Work out the finished part from the listing and answer in its coordinate system (mm). Give positions to 0.01 mm unless a question says otherwise; leave off trailing zeros. Write each loop counter-clockwise with the first axis right and the second up, starting at its lowest first coordinate (ties: lowest second). Pieces come first, ordered by that corner, then holes.
1) Given pin 1 Ø1.5 at (x, z) = (13, -56.5) entering from +Y; pin 2 Ø2 at (x, y) = (12, -6) entering from +Z; pin 3 Ø5 at (x, y) = (2, -7) entering from -Z, each flat-ended and moving along its own axis, determine where each tip first touches the part or whether it passes through.
2) Straight lines are drawn through the part: probe 1 along X at (y, z) = (-20.5, -8); probe 2 along Y at (x, z) = (5, -39.5); probe 3 along X at (y, z) = (-23, -27.5). For each, find the intervals that lie inside material, in ascending order.
3) Find section B-B (y = -9.25). Determine the outline of the cut face in (x, z), plus the area to 3 significant figures.
4) Find section A-A (z = -16). Determine the outline of the cut face in (x, y).
```python
from build123d import *

# Parameters (mm, degrees)
F0_W         = 14.6878659725
F0_H         = 93.4034362435
F1_DEPTH     = 25.4
F2_R         = 5.08
F3_R         = 5.08
F4_T1_DEPTH  = 4.5278659725
F4_T3_DEPTH  = 15.24
F4_S7_W      = 5.08
F4_S7_H      = 5.08
F4_T8_DEPTH  = 5.08
F4_S13_W     = 5.08
F4_S13_H     = 5.08
F4_T14_DEPTH = 5.08
F4_S19_W     = 5.08
F4_S19_H     = 5.08
F4_T20_DEPTH = 5.08
F4_S25_W     = 5.08
F4_S25_H     = 5.08
F4_T26_DEPTH = 5.08
F4_T30_ANGLE = 90
F4_T32_ANGLE = 90
F4_T34_ANGLE = 90
F4_T36_ANGLE = 90


# Not quite as in the source:
# - a fillet or chamfer that OpenCascade refuses, or shapes differently, is made with other operations: its cross-section is extruded or revolved along the edge and cut away or added


with BuildPart() as f1:
    # F0 (on Front) → F1 (new body)
    with BuildSketch(Plane.XZ):
        with Locations((7.3439329863, -46.7017181218)):
            Rectangle(F0_W, F0_H)
    extrude(amount=F1_DEPTH)

    # F2
    f2_edges = [f1.edges().sort_by_distance(p)[0] for p in [
        (14.687866, -25.4, -46.701718),
        (7.343933, -25.4, 0),
        (0, -25.4, -46.701718),
        (7.343933, -25.4, -93.403436),
    ]]
    fillet(f2_edges, radius=F2_R)

    # F3
    f3_edges = [f1.edges().sort_by_distance(p)[0] for p in [
        (14.687866, 0, -46.701718),
        (0, 0, -46.701718),
    ]]
    fillet(f3_edges, radius=F3_R)

    # F4: fillet of radius 5.08 on 2 edges, made by hand

    # F4_s2 → F4_t1 (cut)
    with BuildSketch(Plane.YZ.offset(5.08)):
        with BuildLine():
            ThreePointArc((0, -88.3234362435), (-1.4878975516, -91.915538692), (-5.08, -93.4034362435))
            Line((-5.08, -93.4034362435), (0, -93.4034362435))
            Line((0, -93.4034362435), (0, -88.3234362435))
        make_face()
        with BuildLine():
            ThreePointArc((-5.08, 0), (-1.4878975516, -1.4878975516), (0, -5.08))
            Line((0, -5.08), (0, 0))
            Line((0, 0), (-5.08, 0))
        make_face()
    extrude(amount=F4_T1_DEPTH, mode=Mode.SUBTRACT)

    # F4_s4 → F4_t3 (cut)
    with BuildSketch(Plane.XZ.offset(5.08)):
        with BuildLine():
            ThreePointArc((5.08, 0), (1.4878975516, -1.4878975516), (0, -5.08))
            Line((0, -5.08), (0, 0))
            Line((0, 0), (5.08, 0))
        make_face()
        with BuildLine():
            ThreePointArc((9.6078659725, 0), (13.1999684209, -1.4878975516), (14.6878659725, -5.08))
            Line((14.6878659725, -5.08), (14.6878659725, 0))
            Line((14.6878659725, 0), (9.6078659725, 0))
        make_face()
        with BuildLine():
            ThreePointArc((14.6878659725, -88.3234362435), (13.1999684209, -91.915538692), (9.6078659725, -93.4034362435))
            Line((9.6078659725, -93.4034362435), (14.6878659725, -93.4034362435))
            Line((14.6878659725, -93.4034362435), (14.6878659725, -88.3234362435))
        make_face()
        with BuildLine():
            ThreePointArc((0, -88.3234362435), (1.4878975516, -91.915538692), (5.08, -93.4034362435))
            Line((5.08, -93.4034362435), (0, -93.4034362435))
            Line((0, -93.4034362435), (0, -88.3234362435))
        make_face()
    extrude(amount=F4_T3_DEPTH, mode=Mode.SUBTRACT)


with BuildPart() as f4_tool6:
    # F4_s7 → F4_t8 (new body)
    with BuildSketch(Plane.XY.offset(-5.08)):
        with Locations((2.54, -22.86)):
            Rectangle(F4_S7_W, F4_S7_H)
    extrude(amount=F4_T8_DEPTH)

    # F4_s9 → F4_t10 (revolve, cut)
    with BuildSketch(Plane(origin=(5.08, -20.32, -5.08), x_dir=(0.7071067812, 0.7071067812, 0), z_dir=(0.7071067812, -0.7071067812, 0))):
        with BuildLine():
            ThreePointArc((0, -5.08), (5.08, 0), (0, 5.08))
            Line((0, 5.08), (0, -5.08))
        make_face()
    revolve(axis=Axis((5.08, -20.32, -5.08), (0, 0, 1)), mode=Mode.SUBTRACT)


with BuildPart() as f1_1:
    add(f1.part)

    # F4_t5: cut F4_tool6
    add(f4_tool6.part, mode=Mode.SUBTRACT)


with BuildPart() as f4_tool12:
    # F4_s13 → F4_t14 (new body)
    with BuildSketch(Plane.XY.offset(-5.08)):
        with Locations((12.1478659725, -22.86)):
            Rectangle(F4_S13_W, F4_S13_H)
    extrude(amount=F4_T14_DEPTH)

    # F4_s15 → F4_t16 (revolve, cut)
    with BuildSketch(Plane(origin=(9.6078659725, -20.32, -5.08), x_dir=(-0.7071067812, 0.7071067812, 0), z_dir=(0.7071067812, 0.7071067812, 0))):
        with BuildLine():
            ThreePointArc((0, -5.08), (5.08, 0), (0, 5.08))
            Line((0, 5.08), (0, -5.08))
        make_face()
    revolve(axis=Axis((9.6078659725, -20.32, -5.08), (0, 0, 1)), mode=Mode.SUBTRACT)


with BuildPart() as f1_2:
    add(f1_1.part)

    # F4_t11: cut F4_tool12
    add(f4_tool12.part, mode=Mode.SUBTRACT)


with BuildPart() as f4_tool18:
    # F4_s19 → F4_t20 (new body)
    with BuildSketch(Plane.YZ.offset(9.6078659725)):
        with Locations((-22.86, -90.8634362435)):
            Rectangle(F4_S19_W, F4_S19_H)
    extrude(amount=F4_T20_DEPTH)

    # F4_s21 → F4_t22 (revolve, cut)
    with BuildSketch(Plane(origin=(9.6078659725, -20.32, -88.3234362435), x_dir=(0, 0.7071067812, 0.7071067812), z_dir=(0, 0.7071067812, -0.7071067812))):
        with BuildLine():
            ThreePointArc((0, -5.08), (5.08, 0), (0, 5.08))
            Line((0, 5.08), (0, -5.08))
        make_face()
    revolve(axis=Axis((9.6078659725, -20.32, -88.3234362435), (1, 0, 0)), mode=Mode.SUBTRACT)


with BuildPart() as f1_3:
    add(f1_2.part)

    # F4_t17: cut F4_tool18
    add(f4_tool18.part, mode=Mode.SUBTRACT)


with BuildPart() as f4_tool24:
    # F4_s25 → F4_t26 (new body)
    with BuildSketch(Plane.YZ.offset(5.08)):
        with Locations((-22.86, -90.8634362435)):
            Rectangle(F4_S25_W, F4_S25_H)
    extrude(amount=-F4_T26_DEPTH)

    # F4_s27 → F4_t28 (revolve, cut)
    with BuildSketch(Plane(origin=(5.08, -20.32, -88.3234362435), x_dir=(0, 0.7071067812, 0.7071067812), z_dir=(0, -0.7071067812, 0.7071067812))):
        with BuildLine():
            ThreePointArc((0, -5.08), (5.08, 0), (0, 5.08))
            Line((0, 5.08), (0, -5.08))
        make_face()
    revolve(axis=Axis((5.08, -20.32, -88.3234362435), (-1, 0, 0)), mode=Mode.SUBTRACT)


with BuildPart() as f1_4:
    add(f1_3.part)

    # F4_t23: cut F4_tool24
    add(f4_tool24.part, mode=Mode.SUBTRACT)

    # F4_s29 → F4_t30 (revolve, cut)
    with BuildSketch(Plane.XZ.offset(5.08)):
        with BuildLine():
            ThreePointArc((9.6078659725, 0), (13.1999684209, -1.4878975516), (14.6878659725, -5.08))
            Line((14.6878659725, -5.08), (14.6878659725, 0))
            Line((14.6878659725, 0), (9.6078659725, 0))
        make_face()
    revolve(axis=Axis((9.6078659725, -5.08, 0), (0, 0, 1)), revolution_arc=F4_T30_ANGLE, mode=Mode.SUBTRACT)

    # F4_s31 → F4_t32 (revolve, cut)
    with BuildSketch(Plane.YZ.offset(5.08)):
        with BuildLine():
            ThreePointArc((-5.08, 0), (-1.4878975516, -1.4878975516), (0, -5.08))
            Line((0, -5.08), (0, 0))
            Line((0, 0), (-5.08, 0))
        make_face()
    revolve(axis=Axis((5.08, -5.08, 0), (0, 0, 1)), revolution_arc=F4_T32_ANGLE, mode=Mode.SUBTRACT)

    # F4_s33 → F4_t34 (revolve, cut)
    with BuildSketch(Plane.YZ.offset(5.08)):
        with BuildLine():
            ThreePointArc((0, -88.3234362435), (-1.4878975516, -91.915538692), (-5.08, -93.4034362435))
            Line((-5.08, -93.4034362435), (0, -93.4034362435))
            Line((0, -93.4034362435), (0, -88.3234362435))
        make_face()
    revolve(axis=Axis((5.08, -5.08, -93.4034362435), (0, 0, 1)), revolution_arc=F4_T34_ANGLE, mode=Mode.SUBTRACT)

    # F4_s35 → F4_t36 (revolve, cut)
    with BuildSketch(Plane.XZ.offset(5.08)):
        with BuildLine():
            ThreePointArc((14.6878659725, -88.3234362435), (13.1999684209, -91.915538692), (9.6078659725, -93.4034362435))
            Line((9.6078659725, -93.4034362435), (14.6878659725, -93.4034362435))
            Line((14.6878659725, -93.4034362435), (14.6878659725, -88.3234362435))
        make_face()
    revolve(axis=Axis((9.6078659725, -5.08, -93.4034362435), (0, 0, 1)), revolution_arc=F4_T36_ANGLE, mode=Mode.SUBTRACT)


solid = f1_4.part
```
Results:
1. pin 1: stops at y = -0.74
1. pin 2: stops at z = -0.19
1. pin 3: stops at z = -93.37
2. probe 1: x = 0 to 14.68
2. probe 2: y = -25.4 to 0
2. probe 3: x = 0.76 to 13.92
3. outline: (0, -88.32) arc R5.08 ccw to (5.08, -93.4) - (9.61, -93.4) arc R5.08 ccw to (14.69, -88.32) - (14.69, -5.08) arc R5.08 ccw to (9.61, 0) - (5.08, 0) arc R5.08 ccw to (0, -5.08) - close
3. area: 1,350 mm2
4. outline: (0, -20.32) arc R5.08 ccw to (5.08, -25.4) - (9.61, -25.4) arc R5.08 ccw to (14.69, -20.32) - (14.69, -5.08) arc R5.08 ccw to (9.61, 0) - (5.08, 0) arc R5.08 ccw to (0, -5.08) - close
